Geometry: final body of the model. Coordinates: model frame, mm. Give positions to 0.01 mm unless a question says otherwise; leave off trailing zeros. Order: outer loops, then holes, each group sorted by start corner. A loop starts at its lowest first (then second) coordinate and runs counter-clockwise, first axis right, second up. Notation, with made-up numbers: (-22, 51.25) - (-18, 51.25) arc R14 ccw to (-18, 58.25) - close; hole circle Ø2 at (36, 24.25). An arc over 180 degrees is marked (long way). One line per item, written item: value.
```python
from build123d import *

# Parameters (mm, degrees)
BOSS_EXTRUDE1_DEPTH           = 2
M2_CLEARANCE_HOLE1_D          = 2
M2_CLEARANCE_HOLE1_DEPTH      = 2
M2_CLEARANCE_HOLE1_TIP        = 0.600860619
M3_CLEARANCE_HOLE1_D          = 3
M3_CLEARANCE_HOLE2_D          = 3
M3_CLEARANCE_HOLE2_DEPTH      = 2
M3_CLEARANCE_HOLE2_TIP        = 0.901290929
M3_CLEARANCE_HOLE3_D          = 3
M3_CLEARANCE_HOLE3_DEPTH      = 2
M3_CLEARANCE_HOLE3_TIP        = 0.901290929
FILLET1_R                     = 10
FILLET2_R                     = 10
FILLET3_R                     = 10
FILLET4_R                     = 10
M14_CLEARANCE_HOLE1_D         = 15
M3_CLEARANCE_HOLE4_AT_2_COUNT = 2
M3_CLEARANCE_HOLE4_AT_2_PITCH = 16
M3_CLEARANCE_HOLE4_AT_3_COUNT = 2
M3_CLEARANCE_HOLE4_AT_3_PITCH = 22.627416998
M3_CLEARANCE_HOLE4_AT_4_COUNT = 2
M3_CLEARANCE_HOLE4_AT_4_PITCH = 16
LPATTERN1_COUNT               = 2
LPATTERN1_PITCH               = 94.5


with BuildPart() as part:
    # Sketch1 → Boss-Extrude1 (new body)
    with BuildSketch(Plane(origin=(0, 0, 0), x_dir=(1, 0, 0), z_dir=(0, 1, 0))):
        Polygon((98, 45), (136, 45), (136, 0), (98, 0), (98, -17.5), (38, -17.5), (38, 0), (0, 0), (0, 45), (38, 45), (38, 62.5), (98, 62.5), align=None)
    extrude(amount=BOSS_EXTRUDE1_DEPTH)

    # M2 Clearance Hole1
    with Locations(Plane(origin=(0, 2, 0), x_dir=(1, 0, 0), z_dir=(0, 1, 0))):
        with Locations((2.5, 5), (2.5, 40), (133.5, 40), (133.5, 5)):
            Hole(M2_CLEARANCE_HOLE1_D / 2, depth=M2_CLEARANCE_HOLE1_DEPTH)
            with Locations((0, 0, -(M2_CLEARANCE_HOLE1_DEPTH + M2_CLEARANCE_HOLE1_TIP / 2))):  # 118° drill point
                Cone(0, M2_CLEARANCE_HOLE1_D / 2, M2_CLEARANCE_HOLE1_TIP, mode=Mode.SUBTRACT)

    # M3 Clearance Hole1 (through all)
    with Locations(Plane(origin=(0, 2, 0), x_dir=(1, 0, 0), z_dir=(0, 1, 0))):
        with Locations((41.5, 39), (94.5, 39), (94.5, -14), (41.5, -14)):
            Hole(M3_CLEARANCE_HOLE1_D / 2)

    # M3 Clearance Hole2
    with Locations(Plane(origin=(0, 2, 0), x_dir=(1, 0, 0), z_dir=(0, 1, 0))):
        with Locations((41.5, -4), (94.5, -4), (94.5, 49), (41.5, 49)):
            Hole(M3_CLEARANCE_HOLE2_D / 2, depth=M3_CLEARANCE_HOLE2_DEPTH)
            with Locations((0, 0, -(M3_CLEARANCE_HOLE2_DEPTH + M3_CLEARANCE_HOLE2_TIP / 2))):  # 118° drill point
                Cone(0, M3_CLEARANCE_HOLE2_D / 2, M3_CLEARANCE_HOLE2_TIP, mode=Mode.SUBTRACT)

    # M3 Clearance Hole3
    with Locations(Plane(origin=(0, 2, 0), x_dir=(1, 0, 0), z_dir=(0, 1, 0))):
        with Locations((41.5, 59), (94.5, 59), (94.5, 6), (41.5, 6)):
            Hole(M3_CLEARANCE_HOLE3_D / 2, depth=M3_CLEARANCE_HOLE3_DEPTH)
            with Locations((0, 0, -(M3_CLEARANCE_HOLE3_DEPTH + M3_CLEARANCE_HOLE3_TIP / 2))):  # 118° drill point
                Cone(0, M3_CLEARANCE_HOLE3_D / 2, M3_CLEARANCE_HOLE3_TIP, mode=Mode.SUBTRACT)

    # Fillet1
    fillet1_edges = [part.edges().sort_by_distance(p)[0] for p in [
        (98, 1, 0),
    ]]
    fillet(fillet1_edges, radius=FILLET1_R)

    # Fillet2
    fillet2_edges = [part.edges().sort_by_distance(p)[0] for p in [
        (98, 1, -45),
    ]]
    fillet(fillet2_edges, radius=FILLET2_R)

    # Fillet3
    fillet3_edges = [part.edges().sort_by_distance(p)[0] for p in [
        (38, 1, 0),
    ]]
    fillet(fillet3_edges, radius=FILLET3_R)

    # Fillet4
    fillet4_edges = [part.edges().sort_by_distance(p)[0] for p in [
        (38, 1, -45),
    ]]
    fillet(fillet4_edges, radius=FILLET4_R)

    # M14 Clearance Hole1 (through all)
    with Locations(Plane(origin=(0, 2, 0), x_dir=(1, 0, 0), z_dir=(0, 1, 0))):
        with Locations((115.25, 22.5), (20.75, 22.5)):
            Hole(M14_CLEARANCE_HOLE1_D / 2)

    # Sketch14 → M3 Clearance Hole4 (revolve, cut)
    with BuildSketch(Plane(origin=(107.25, 2, -30.5), x_dir=(0, 0, 1), z_dir=(1, 0, 0))):
        Polygon((0, 0), (0, 2.901290929), (1.5, 2), (1.5, 0), align=None)
    m3_clearance_hole4 = revolve(axis=Axis((107.25, 8.35, -30.5), (0, -1, 0)), mode=Mode.SUBTRACT)

    # M3 Clearance Hole4 at 2: M3 Clearance Hole4 ×2
    with Locations(*[(i * M3_CLEARANCE_HOLE4_AT_2_PITCH, 0, 0) for i in range(1, M3_CLEARANCE_HOLE4_AT_2_COUNT)]):
        add(m3_clearance_hole4, mode=Mode.SUBTRACT)

    # M3 Clearance Hole4 at 3: M3 Clearance Hole4 ×2
    with Locations(*[Vector(0.7071067811865472, 0, 0.7071067811865479) * (i * M3_CLEARANCE_HOLE4_AT_3_PITCH) for i in range(1, M3_CLEARANCE_HOLE4_AT_3_COUNT)]):
        add(m3_clearance_hole4, mode=Mode.SUBTRACT)

    # M3 Clearance Hole4 at 4: M3 Clearance Hole4 ×2
    with Locations(*[(0, 0, i * M3_CLEARANCE_HOLE4_AT_4_PITCH) for i in range(1, M3_CLEARANCE_HOLE4_AT_4_COUNT)]):
        add(m3_clearance_hole4, mode=Mode.SUBTRACT)

    # LPattern1: M3 Clearance Hole4 ×2
    with Locations(*[(-i * LPATTERN1_PITCH, 0, 0) for i in range(1, LPATTERN1_COUNT)]):
        add(m3_clearance_hole4, mode=Mode.SUBTRACT)

    # LPattern1 copy 1 sketch → LPattern1 copy 1 (revolve, cut)
    with BuildSketch(Plane(origin=(28.75, 2, -30.5), x_dir=(0, 0, 1), z_dir=(1, 0, 0))):
        Polygon((0, 0), (0, 2.901290929), (1.5, 2), (1.5, 0), align=None)
    revolve(axis=Axis((28.75, 8.35, -30.5), (0, -1, 0)), mode=Mode.SUBTRACT)

    # LPattern1 copy 2 sketch → LPattern1 copy 2 (revolve, cut)
    with BuildSketch(Plane(origin=(28.75, 2, -14.5), x_dir=(0, 0, 1), z_dir=(1, 0, 0))):
        Polygon((0, 0), (0, 2.901290929), (1.5, 2), (1.5, 0), align=None)
    revolve(axis=Axis((28.75, 8.35, -14.5), (0, -1, 0)), mode=Mode.SUBTRACT)

    # LPattern1 copy 3 sketch → LPattern1 copy 3 (revolve, cut)
    with BuildSketch(Plane(origin=(12.75, 2, -14.5), x_dir=(0, 0, 1), z_dir=(1, 0, 0))):
        Polygon((0, 0), (0, 2.901290929), (1.5, 2), (1.5, 0), align=None)
    revolve(axis=Axis((12.75, 8.35, -14.5), (0, -1, 0)), mode=Mode.SUBTRACT)


solid = part.part
```
1) Section C-C, the plane x = 94.5. Return loops of the section in (y, z), then the cut area to 3 significant figures.
Answers below:
outline: (0, -62.5) - (2, -62.5) - (2, -60.5) - (0, -60.5) - close; (0, -57.5) - (2, -57.5) - (2, -50.5) - (0, -50.5) - close; (0, -47.5) - (2, -47.5) - (2, -40.5) - (0, -40.5) - close; (0, -37.5) - (2, -37.5) - (2, -7.5) - (0, -7.5) - close; (0, -4.5) - (2, -4.5) - (2, 2.5) - (0, 2.5) - close; (0, 5.5) - (2, 5.5) - (2, 12.5) - (0, 12.5) - close; (0, 15.5) - (2, 15.5) - (2, 17.5) - (0, 17.5) - close
area: 124 mm^2
2) Section A-A, the plane x = 20.75. Return loops of the section in (y, z).
Answers below:
outline: (0, -45) - (2, -45) - (2, -30) - (0, -30) - close; (0, -15) - (2, -15) - (2, 0) - (0, 0) - close
3) Section B-B, the plane z = -49. Return loops of the section in (x, y), then the cut area to 3 significant figures.
Answers below:
outline: (36, 0) - (40, 0) - (40, 2) - (36, 2) - close; (43, 0) - (93, 0) - (93, 2) - (43, 2) - close; (96, 0) - (100, 0) - (100, 2) - (96, 2) - close
area: 116 mm^2
4) Mould query, pull axis X, two halves, no side actions, for faces 1 (the face through (34.99, 1.01, -47.85)), 2 (the face through (43, 1, 14)), 3 (the face through (93.81, 0.99, -47.67)), 4 (the face through (69, 0, -23)). Classes: released by +X, released by -X, zero draft, split by the parting line, or undercut.
Answers below:
face 1: released by -X
face 2: undercut
face 3: undercut
face 4: zero draft
5) Section D-D, the plane y = 0.3. Count the separate pieces of the cut face and the enclosed holes in it, then the cut area to 3 significant figures.
Answers below:
separate pieces: 1
enclosed holes: 26
area: 7,800 mm^2
6) First-contact query: pin 1 (1.8 mm diameter, centred on x = 41.5, z = -6, fed in from +Y); pin 2 (0.6 mm diameter, centred on x = 128.5, y = 1, fed in from -Z); pin 3 (1 mm diameter, centred on y = 1.5, z = -58.5, fed in from -X). Flat tips, straight axial feed; report the tip coordinate or a pass-through.
Answers below:
pin 1: through
pin 2: z = -45
pin 3: x = 38
7) Material intervals for line 1 along Z through (x, y) = (2.5, 1.45); line 2 along Z through (x, y) = (28.75, 1.35); line 3 along X through (y, z) = (1.35, -30.5), sorted ascending.
Answers below:
line 1: -45 to -41, -39 to -6, -4 to 0
line 2: -45.03 to -32, -29 to -16, -13 to 0.03
line 3: 0 to 11.25, 14.25 to 27.25, 30.25 to 105.75, 108.75 to 121.75, 124.75 to 136
